from build123d import *

# Parameters (mm, degrees)
F0_W     = 8
F0_H     = 4
F0_W_2   = 5
F0_H_2   = 6
F0_W_3   = 15.5
F0_H_3   = 13
F1_DEPTH = 1.8
F2_DEPTH = 2
F3_DEPTH = 2


# Not quite as in the source:
# - a feature of the source that left no trace in its solid (it failed there, or was rolled back) is left out


with BuildPart() as f1:
    # F0 (on Front) → F1 (new body)
    with BuildSketch(Plane.XZ):
        with BuildLine():
            Line((34.7865003794, 6.2641621617), (-29.2134996206, 6.2641621617))
            ThreePointArc((-29.2134996206, 6.2641621617), (-31.3348199641, 5.3854825052), (-32.2134996206, 3.2641621617))
            Line((-32.2134996206, 3.2641621617), (-32.2134996206, -19.6358378383))
            ThreePointArc((-32.2134996206, -19.6358378383), (-31.3348199641, -21.7571581819), (-29.2134996206, -22.6358378383))
            Line((-29.2134996206, -22.6358378383), (34.7865003794, -22.6358378383))
            ThreePointArc((34.7865003794, -22.6358378383), (36.907820723, -21.7571581819), (37.7865003794, -19.6358378383))
            Line((37.7865003794, -19.6358378383), (37.7865003794, 3.2641621617))
            ThreePointArc((37.7865003794, 3.2641621617), (36.907820723, 5.3854825052), (34.7865003794, 6.2641621617))
        make_face()
        with Locations((-0.6956385732, -12.2858378383)):
            Rectangle(F0_W, F0_H, mode=Mode.SUBTRACT)
        with Locations((14.8043614268, -9.3358378383)):
            Rectangle(F0_W_2, F0_H_2, mode=Mode.SUBTRACT)
        with Locations((25.3043614268, -9.3358378383)):
            Rectangle(F0_W_2, F0_H_2, mode=Mode.SUBTRACT)
        with Locations((-15.8456385732, -7.7858378383)):
            Rectangle(F0_W_3, F0_H_3, mode=Mode.SUBTRACT)
    extrude(amount=F1_DEPTH)

    # F0 (on Front) → F2 (join)
    with BuildSketch(Plane.XZ):
        with BuildLine():
            Line((34.7865003794, 6.2641621617), (-29.2134996206, 6.2641621617))
            ThreePointArc((-29.2134996206, 6.2641621617), (-31.3348199641, 5.3854825052), (-32.2134996206, 3.2641621617))
            Line((-32.2134996206, 3.2641621617), (-32.2134996206, -19.6358378383))
            ThreePointArc((-32.2134996206, -19.6358378383), (-31.3348199641, -21.7571581819), (-29.2134996206, -22.6358378383))
            Line((-29.2134996206, -22.6358378383), (34.7865003794, -22.6358378383))
            ThreePointArc((34.7865003794, -22.6358378383), (36.907820723, -21.7571581819), (37.7865003794, -19.6358378383))
            Line((37.7865003794, -19.6358378383), (37.7865003794, 3.2641621617))
            ThreePointArc((37.7865003794, 3.2641621617), (36.907820723, 5.3854825052), (34.7865003794, 6.2641621617))
        make_face()
        with Locations((-0.6956385732, -12.2858378383)):
            Rectangle(F0_W, F0_H, mode=Mode.SUBTRACT)
        with Locations((14.8043614268, -9.3358378383)):
            Rectangle(F0_W_2, F0_H_2, mode=Mode.SUBTRACT)
        with Locations((25.3043614268, -9.3358378383)):
            Rectangle(F0_W_2, F0_H_2, mode=Mode.SUBTRACT)
        with Locations((-15.8456385732, -7.7858378383)):
            Rectangle(F0_W_3, F0_H_3, mode=Mode.SUBTRACT)
    extrude(amount=F2_DEPTH)

    # F3 (add): a face of the model
    f3_faces = [f1.faces().sort_by_distance(p)[0] for p in [
        (4.4299984424, -2, -8.1163746121),
    ]]
    extrude(f3_faces, amount=F3_DEPTH)


solid = f1.part
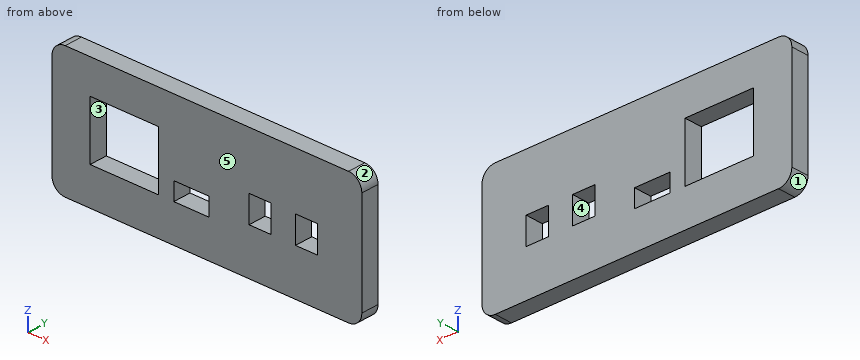
Geometry check sheet. Reference: the model listing, model coordinates, mm. Face numbers are marked on the shaded views. A direction names the side the tool comes from. Coordinates: 2 decimals unless noted, no trailing zeros. Order: outer loops, then holes, each group sorted by start corner. A loop starts at its lowest first (then second) coordinate and runs counter-clockwise, first axis right, second up. Notation, with made-up numbers: (45, 38) -> (50, 38) arc R18 ccw to (50, 52) -> close; hole circle Ø5 at (21.5, -7.5). An arc over 180 degrees is marked (long way). Use a Markdown table: item, result. Add a question column.
1. Cross-section at D-D (y = -1.4). Enter the section's corners in (x, z), and give its area (3 significant figures).
2. Cross-section at C-C (z = -3.75). Enter the section's corners in (x, y).
3. Cross-section at B-B (z = -13). Enter the section's corners in (x, y).
4. Cross-section at A-A (x = 13). Enter the section's corners in (y, z), and give its area (3 significant figures).
5. Material ranges on L1, parallel to X at y = -3.8, z = -8.5; L2, parallel to X at y = -3.8, z = -12.25; L3, parallel to Z at x = -9, y = -2.7, recorded low to high.
6. Mould release check, pull along Z, two halves, no side actions. Record for the marked faces 1, 2 and 3: pulls with the +Z half, pulls with the -Z half, needs draft (parallel to the pull), parting line crosses it, or undercut.
7. Set-up check for the marked faces 4 and 5: record each of +Z, -Z, +X, -X, +Y, -Y from which the full face is reachable in a straight line by a thin tool's end or side.
Filled sheet:
| question | item | result |
|---|---|---|
| 1 | outline | (-32.21, -19.64) arc R3 ccw to (-29.21, -22.64) -> (34.79, -22.64) arc R3 ccw to (37.79, -19.64) -> (37.79, 3.26) arc R3 ccw to (34.79, 6.26) -> (-29.21, 6.26) arc R3 ccw to (-32.21, 3.26) -> close; hole (-23.6, -14.29) -> (-8.1, -14.29) -> (-8.1, -1.29) -> (-23.6, -1.29) -> close; hole (-4.7, -14.29) -> (3.3, -14.29) -> (3.3, -10.29) -> (-4.7, -10.29) -> close; hole (12.3, -12.34) -> (17.3, -12.34) -> (17.3, -6.34) -> (12.3, -6.34) -> close; hole (22.8, -12.34) -> (27.8, -12.34) -> (27.8, -6.34) -> (22.8, -6.34) -> close |
| 1 | area | 1,720 mm2 |
| 2 | outline | (-32.21, -4) -> (-23.6, -4) -> (-23.6, 0) -> (-32.21, 0) -> close; (-8.1, -4) -> (37.79, -4) -> (37.79, 0) -> (-8.1, 0) -> close |
| 3 | outline | (-32.21, -4) -> (-23.6, -4) -> (-23.6, 0) -> (-32.21, 0) -> close; (-8.1, -4) -> (-4.7, -4) -> (-4.7, 0) -> (-8.1, 0) -> close; (3.3, -4) -> (37.79, -4) -> (37.79, 0) -> (3.3, 0) -> close |
| 4 | outline | (-4, -22.64) -> (0, -22.64) -> (0, -12.34) -> (-4, -12.34) -> close; (-4, -6.34) -> (0, -6.34) -> (0, 6.26) -> (-4, 6.26) -> close |
| 4 | area | 91.6 mm2 |
| 5 | L1 | -32.21 to -23.6, -8.1 to 12.3, 17.3 to 22.8, 27.8 to 37.79 |
| 5 | L2 | -32.21 to -23.6, -8.1 to -4.7, 3.3 to 12.3, 17.3 to 22.8, 27.8 to 37.79 |
| 5 | L3 | -22.64 to -14.29, -1.29 to 6.26 |
| 6 | face 1 | pulls with the -Z half |
| 6 | face 2 | pulls with the +Z half |
| 6 | face 3 | undercut |
| 7 | face 4 | +Y, -Y |
| 7 | face 5 | +Z, -Z, +X, -X, -Y |
